Work out the finished part from the listing and answer in its coordinate system (mm). A direction names the side the tool comes from. Round coordinates to 2 decimals unless told otherwise and drop trailing zeros. Write each loop counter-clockwise with the first axis right and the second up, starting at its lowest first coordinate (ties: lowest second). Pieces come first, ordered by that corner, then holes. Notation, with made-up numbers: M 52.25,74 L 67.25,74 A37 cw 67.25,113 Z; hole C 71,-14 d8. An arc over 180 degrees is marked long. Answer in a Markdown table with one row per item.
```python
from build123d import *

# Parameters (mm, degrees)
F0_W      = 35.91213
F0_H      = 41.681683
F1_DEPTH  = 7.112
F2_W      = 4.138863
F2_H      = 3.556104
F3_DEPTH  = 99.06
F4_W      = 4.138863
F4_H      = 3.091657
F5_DEPTH  = 100.584
F6_W      = 3.981255
F6_H      = 5.324956
F7_DEPTH  = 100.584
F8_W      = 5.462058
F8_H      = 3.072897
F9_DEPTH  = 100.33
F10_W     = 3.054641
F10_H     = 41.681683
F11_DEPTH = 68.072


with BuildPart() as f1:
    # F0 (on Top) → F1 (new body)
    with BuildSketch(Plane.XY):
        with Locations((-43.722132, -7.864382)):
            Rectangle(F0_W, F0_H)
    extrude(amount=F1_DEPTH)

    # F2 (on face) → F3 (join)
    with BuildSketch(Plane(origin=(0, 0, 0), x_dir=(1, 0, 0), z_dir=(0, 0, -1))):
        with Locations((-27.835498, 25.163998)):
            Rectangle(F2_W, F2_H)
    extrude(amount=F3_DEPTH)

    # F4 (on face) → F5 (join)
    with BuildSketch(Plane(origin=(0, 0, 0), x_dir=(1, 0, 0), z_dir=(0, 0, -1))):
        with Locations((-27.835498, -8.937603)):
            Rectangle(F4_W, F4_H)
    extrude(amount=F5_DEPTH)

    # F6 (on face) → F7 (join)
    with BuildSketch(Plane(origin=(0, 0, 0), x_dir=(1, 0, 0), z_dir=(0, 0, -1))):
        with Locations((-59.687569, -10.313982)):
            Rectangle(F6_W, F6_H)
    extrude(amount=F7_DEPTH)

    # F8 (on face) → F9 (join)
    with BuildSketch(Plane(origin=(0, 0, 0), x_dir=(1, 0, 0), z_dir=(0, 0, -1))):
        with Locations((-58.947168, 24.504973)):
            Rectangle(F8_W, F8_H)
    extrude(amount=F9_DEPTH)

    # F10 (on face) → F11 (join)
    with BuildSketch(Plane.XY.offset(7.112)):
        with Locations((-60.150876, -7.864382)):
            Rectangle(F10_W, F10_H)
    extrude(amount=F11_DEPTH)


solid = f1.part
```
1. A tool of negligible diameter and unlimited length cuts with its end or side. For faces 1 (the flat face through (-42, -8, 7.112)), 2 (the flat face through (-28, 10.483, -50)), 3 (the flat face through (-57.697, 10, -50)), 4 (the flat face through (-59, -25, -100.33)), from which of +Z, -Z, +X, -X, +Y, -Y can it reach the whole face along a straight path? Write none if from no direction.
Calculated:
| item | result |
|---|---|
| face 1 | +Z, +X, +Y, -Y |
| face 2 | -Z, +X, +Y |
| face 3 | -Z, +Y |
| face 4 | -Z, +X, -X, -Y |
2. Determine the mould class of faces 5 (the flat face through (-29.905, 9, -50)), 6 (the flat face through (-60, 7.652, -50)), 7 (the flat face through (-25.766, -8, 4)) for opening direction X: released by +X, released by -X, zero draft, split by the parting line, or undercut.
Calculated:
| item | result |
|---|---|
| face 5 | undercut |
| face 6 | zero draft |
| face 7 | released by +X |
3. The part is cut by section C-C (y = -9). Determine the outline of the cut face in (x, z).
Calculated:
| item | result |
|---|---|
| outline | M -61.68,0 L -25.77,0 L -25.77,7.11 L -58.62,7.11 L -58.62,75.18 L -61.68,75.18 Z |
4. Consider line 1 along Y through (x, z) = (-58, -75); line 2 along Z through (x, y) = (-47, 11.5); line 3 along X through (y, z) = (-6.5, 56). Determine where each line is inside the solid, lowest interval first. Write a range as from..to.
Calculated:
| item | result |
|---|---|
| line 1 | y = -26.04..-22.97, 7.65..12.98 |
| line 2 | z = 0..7.11 |
| line 3 | x = -61.68..-58.62 |
5. The part is cut by section D-D (z = 46). Determine the outline of the cut face in (x, y), plus the area to 3 significant figures.
Calculated:
| item | result |
|---|---|
| outline | M -61.68,-28.71 L -58.62,-28.71 L -58.62,12.98 L -61.68,12.98 Z |
| area | 127 mm² |
6. The part is cut by section B-B (x = -28). Determine the outline of the cut face in (y, z), plus the area to 3 significant figures.
Calculated:
| item | result |
|---|---|
| outline | M -28.71,0 L -26.94,0 L -26.94,-99.06 L -23.39,-99.06 L -23.39,0 L 7.39,0 L 7.39,-100.58 L 10.48,-100.58 L 10.48,0 L 12.98,0 L 12.98,7.11 L -28.71,7.11 Z |
| area | 960 mm² |
7. Given pin 1 (10 mm diameter, centred on y = -10, z = 40, fed in from +X); pin 2 (3.5 mm diameter, centred on x = -58, y = -24, fed in from -Z); pin 3 (4.5 mm diameter, centred on x = -27, z = -63, fed in from -Y); pin 4 (10 mm diameter, centred on y = 6, z = -28, fed in from -X), each flat-ended and moving along its own axis, determine where each tip first touches the part or whether it passes through.
Calculated:
| item | result |
|---|---|
| pin 1 | stops at x = -58.62 |
| pin 2 | stops at z = -100.33 |
| pin 3 | stops at y = -26.94 |
| pin 4 | stops at x = -61.68 |
8. The part is cut by section A-A (z = -72). Determine the outline of the cut face in (x, y).
Calculated:
| item | result |
|---|---|
| outline | M -61.68,-26.04 L -56.22,-26.04 L -56.22,-22.97 L -61.68,-22.97 Z; M -61.68,7.65 L -57.7,7.65 L -57.7,12.98 L -61.68,12.98 Z; M -29.9,-26.94 L -25.77,-26.94 L -25.77,-23.39 L -29.9,-23.39 Z; M -29.9,7.39 L -25.77,7.39 L -25.77,10.48 L -29.9,10.48 Z |
